Autodesk Inventor part; units mm, degrees
ref_plane "YZ Plane" through (0, 0, 0) normal (1, 0, 0) x (0, 1, 0)
ref_plane "XZ Plane" through (0, 0, 0) normal (0, 1, 0) x (-1, 0, 0)
ref_plane "XY Plane" through (0, 0, 0) normal (0, 0, 1) x (1, 0, 0)
sketch "Sketch1" plane through (0, 0, 0) normal (1, 0, 0) x (0, 1, 0)
  line L0 (-3.0178, 2.5025) -> (21.9822, 2.5025)
  line L1 (21.9822, 2.5025) -> (21.9822, -3.4975)
  line L2 (21.9822, -3.4975) -> (-3.0178, -3.4975)
  line L3 (-3.0178, -3.4975) -> (-3.0178, 2.5025)
  circle A0 centre (-1.0178, 0.668) radius 0.5
  circle A1 centre (18.9822, 0.668) radius 0.5
  line L4 (16.4822, -3.4975) -> (2.4822, -3.4975)
  line L5 (2.4822, -3.4975) -> (2.4822, -9.4975)
  line L6 (2.4822, -9.4975) -> (16.4822, -9.4975)
  line L7 (9.9822, 2.5025) -> (8.9822, 2.5025)
  line L8 (8.9822, 2.5025) -> (8.9822, 8.5025)
  line L9 (8.9822, 8.5025) -> (9.9822, 8.5025)
  line L10 (9.9822, 8.5025) -> (9.9822, 2.5025)
  line L11 (16.4822, -9.4975) -> (16.4822, -3.4975)
  circle A2 centre (-1.0178, -5.932) radius 0.5
  line L12 (2.4822, -4.5336) -> (-3.0178, -4.5336)
  line L13 (-3.0178, -4.5336) -> (-3.0178, -7.908)
  line L14 (-3.0178, -7.908) -> (2.4822, -7.908)
  line L15 (2.4822, -7.908) -> (2.4822, -4.5336)
  point P0 (0, 0)
  dimension "d0" = 25
  dimension "d1" = 6
  dimension "d2" = 1
  dimension "d3" = 1
  dimension "d4" = 20
  dimension "d5" = 14
  dimension "d6" = 6
  dimension "d8" = 1
  dimension "d9" = 6
  dimension "d10" = 10
  dimension "d13" = 2
  dimension "d18" = 3
  dimension "d19" = 5.5
  dimension "d20" = 1
  dimension "d21" = 6.6
extrude "Extrusion1" add sketch "Sketch1" along normal blind 5
sketch "Sketch2" plane through (0, 8.9822, 2.5025) normal (0, -1, 0) x (1, 0, 0)
  line L0 (0, 6) -> (0, 0)
  line L1 (0, 0) -> (5, 0)
  line L2 (5, 6) -> (5, 0)
  line L3 (0, 6) -> (5, 6)
  circle A0 centre (2.5, 3) radius 0.5
  point P0 (0, -2.5025)
  dimension "d14" = 1
extrude "Extrusion2" cut sketch "Sketch2" against normal blind 5 contours A0
sketch "Skizze3" plane through (0, 21.9822, 2.5025) normal (0, 1, 0) x (1, 0, 0)
  line L0 (0, 0) -> (0, 6)
  line L1 (0, 0) -> (5, 0)
  line L2 (5, 6) -> (5, 0)
  line L3 (0, 6) -> (5, 6)
  line L4 (0, 2.3346) -> (5, 2.3346)
  line L5 (0, 1.3346) -> (5, 1.3346)
  circle A0 centre (3.2995, 1.8094) radius 0.9299
  point P0 (0, 2.5025)
extrude "Extrusion3" cut sketch "Skizze3" against normal blind 10 contours A0 L4 L5 | L5 A0 | A0 L4
properties part number "00_Microlinearmotor"
Can you work these out from the model? Positions are in its coordinate system, mm. A direction names the side the tool comes from. Round coordinates to 2 decimals unless told otherwise and drop trailing zeros. Loops run counter-clockwise (first coordinate to the right, second up) from the corner with the lowest first, then second, coordinate; pieces in that order, holes last. Notation, with made-up numbers: M 58,22 L 113,22 A7 cw 113,35 Z; hole C 84,63.5 d7. An arc over 180 degrees is marked long. Answer as a JSON object with one key per item and string values. Group by question number.
Q1. Imagine slicing it at D-D, the plane y = 14.5. Please give me the cut outline in (x, z), then the cut area to 3 significant figures.
Q2. We'd pull the mould along Z, two halves only. Please class faces 4 (the flat face through (2, 19, -3.498)), 5 (the flat face through (2, 2.482, -9)), 6 (the cylindrical face through (2.465, -1.386, -6.27)), 7 (the cylindrical face through (1.25, 19.46, 0.52)): +Z half, -Z half, draft (parallel to the pull), parting line (faces both ways), or undercut.
Q3. Imagine slicing it at A-A, the plane y = 0.5. Please give me the cut outline in (x, z).
Q4. Imagine slicing it at B-B, the plane x = 4.5. Please give me the cut outline in (y, z).
Q5. Imagine slicing it at C-C, the plane x = 3.4. Please give me the cut outline in (y, z).
Q6. On a 3-axis mill with a long thin cutter (end or side, diameter ignored), from which of +Z, -Z, +X, -X, +Y, -Y can I reach the whole of each face in a straight line? I mean faces 1 (the flat face through (2, 0, -4.534)), 2 (the cylindrical face through (2.37, 17.05, 0.65)), 3 (the flat face through (2, 16.482, -7)). Say none if no direction works.
Q7. Please list where these lines run through material, in increasing order: L1, parallel to Z at x = 3.65, y = 0.5; L2, parallel to Y at x = 2.25, z = 0.5; L3, parallel to Z at x = 0.8, y = -0.75.
Q8. Will these pins go through, and if not, where does the flat tip stop? pin 1 (1.5 mm diameter, centred on x = 2.5, y = 0, fed in from +Z); pin 2 (2.5 mm diameter, centred on x = 1.5, y = 0.5, fed in from -Z); pin 3 (1.5 mm diameter, centred on x = 1.5, z = 5, fed in from -Y).
Findings:
{
 "1": {"outline": "M 0,-9.5 L 5,-9.5 L 5,2.5 L 0,2.5 Z; hole C 3.3,0.69 d1.86", "area": "57.3 mm2"},
 "2": {"face 4": "-Z half", "face 5": "draft", "face 6": "undercut", "face 7": "undercut"},
 "3": {"outline": "M 0,-7.91 L 5,-7.91 L 5,-4.53 L 0,-4.53 Z; M 0,-3.5 L 5,-3.5 L 5,2.5 L 0,2.5 Z"},
 "4": {"outline": "M -3.02,-7.91 L 2.48,-7.91 L 2.48,-9.5 L 16.48,-9.5 L 16.48,-3.5 L 21.98,-3.5 L 21.98,2.5 L 9.98,2.5 L 9.98,8.5 L 8.98,8.5 L 8.98,2.5 L -3.02,2.5 L -3.02,-3.5 L 2.48,-3.5 L 2.48,-4.53 L -3.02,-4.53 Z; hole C -1.02,-5.93 d1; hole C -1.02,0.67 d1; hole C 18.98,0.67 d1"},
 "5": {"outline": "M -3.02,-7.91 L 2.48,-7.91 L 2.48,-9.5 L 16.48,-9.5 L 16.48,-3.5 L 21.98,-3.5 L 21.98,-0.23 L 11.98,-0.23 L 11.98,1.62 L 21.98,1.62 L 21.98,2.5 L 9.98,2.5 L 9.98,8.5 L 8.98,8.5 L 8.98,2.5 L -3.02,2.5 L -3.02,-3.5 L 2.48,-3.5 L 2.48,-4.53 L -3.02,-4.53 Z; hole C -1.02,-5.93 d1; hole C -1.02,0.67 d1"},
 "6": {"face 1": "+X, -X, -Y", "face 2": "+Y", "face 3": "-Z, +X, -X, +Y"},
 "7": {"L1": "z = -7.91 to -4.53, -3.5 to 2.5", "L2": "y = -3.02 to -1.49, -0.55 to 18.51, 19.45 to 21.98", "L3": "z = -7.91 to -6.35, -5.51 to -4.53, -3.5 to 0.25, 1.09 to 2.5"},
 "8": {"pin 1": "stops at z = 2.5", "pin 2": "stops at z = -7.91", "pin 3": "stops at y = 8.98"}
}
